Autodesk Fusion 360 part; units mm, degrees
sketch "Skizze8" plane through (0, 0, 0) normal (1, 0, 0) x (0, 1, 0)
  line L0 (-6.5, 80) -> (-16.5, 80)
  line L1 (-16.5, 80) -> (-16.5, -80)
  line L2 (-16.5, -80) -> (-6.5, -80)
  line L3 (-6.5, -80) -> (-6.5, -30)
  line L4 (3.5, -20) -> (25, -20)
  line L5 (35, -10) -> (35, 0)
  line L6 (25, 10) -> (3.5, 10)
  line L7 (105.6778, -5) -> (-37.6639, -5) construction
  line L8 (25, 49.113) -> (25, -113.6091) construction
  line L9 (-6.5, 20) -> (-6.5, 80)
  arc A0 (-6.5, 20) -> (3.5, 10) centre (3.5, 20) ccw
  arc A1 (3.5, -20) -> (-6.5, -30) centre (3.5, -30) ccw
  arc A2 (35, 0) -> (25, 10) centre (25, 0) ccw
  arc A3 (25, -20) -> (35, -10) centre (25, -10) ccw
  circle A4 centre (25, -5) radius 4.15
  point P0 (-6.5, 10)
  dimension "d127" = 80
  dimension "d128" = 80
  dimension "d129" = 5
  dimension "d130" = 31.5
  dimension "d131" = 25
  dimension "d132" = 10
  dimension "d133" = 10
  dimension "d134" = 15
  dimension "d135" = 15
  dimension "d136" = 10
  dimension "d137" = 10
  dimension "d138" = 10
  dimension "d139" = 10
  dimension "d140" = 10
  dimension "d141" = 10
  dimension "d142" = 8.3
extrude "Extrusion8" add sketch "Skizze8" along normal mid plane 40
sketch "Skizze9" plane through (0, 0, 0) normal (0, 0, 1) x (1, 0, 0)
  line L0 (10.1, 40) -> (-10.1, 40)
  line L1 (-10.1, 40) -> (-10.1, -6.5)
  line L2 (-10.1, -6.5) -> (10.1, -6.5)
  line L3 (10.1, -6.5) -> (10.1, 40)
  dimension "d145" = 6.5
  dimension "d146" = 40
  dimension "d147" = 10.1
  dimension "d148" = 10.1
extrude "Extrusion9" cut sketch "Skizze9" along normal mid plane 200
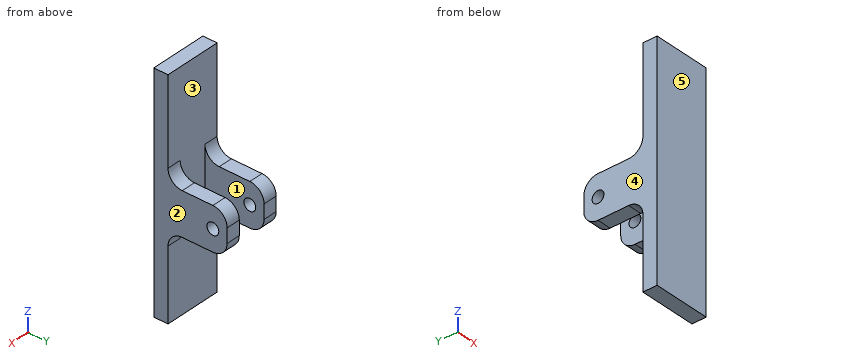
Geometry: final body of the model. Coordinates: model frame, mm. Face numbers are marked on the shaded views. A direction names the side the tool comes from. Round coordinates to 2 decimals unless told otherwise and drop trailing zeros. Write each loop counter-clockwise with the first axis right and the second up, starting at its lowest first coordinate (ties: lowest second). Pieces come first, ordered by that corner, then holes. Notation, with made-up numbers: (46, 30) -> (62, 30) arc R30 ccw to (62, 59) -> close; hole circle Ø6 at (34, -20). An arc over 180 degrees is marked (long way). Use CSV: the item, a comma, the result in double quotes. Start each with the question number.
Q1. Section B-B (y = 11). Return loops of the section in (x, z).
Q2. Section A-A (z = -5). Return loops of the section in (x, y), plus the area to 3 significant figures.
Q3. Section D-D (x = -7.5). Return loops of the section in (y, z), plus the area to 3 significant figures.
Q4. First-contact query: pin 1 Ø11 at (x, y) = (-15, 18.5) entering from +Z; pin 2 Ø7.5 at (y, z) = (25, -5) entering from +X; pin 3 Ø10 at (x, z) = (12, 18) entering from +Y; pin 4 Ø3 at (x, y) = (-16, 10) entering from -Z. Flat tips, straight axial feed; report the tip coordinate or a pass-through.
Q5. Section C-C (x = 11.5). Return loops of the section in (y, z), plus the area to 3 significant figures.
Q6. Pull-direction query (X, two-part tool) for the marked faces 3, 4 and 5; classes: pulls with the +X half, pulls with the -X half, needs draft (parallel to the pull), parting line crosses it, or undercut.
Q7. Reachability of the marked faces 1 and 2 from +Z, -Z, +X, -X, +Y, -Y: full face, straight path, thin tool, end or side. Return the list, or none.
Q8. Line query: L1, parallel to Z at x = -15.5, y = 25; L2, parallel to Y at x = 13, z = -5; L3, parallel to Y at x = -9, z = -6.5. Output: solid intervals per line, ascending.
Result sheet:
1,outline,"(-20, -20) -> (-10.1, -20) -> (-10.1, 10) -> (-20, 10) -> close; (10.1, -20) -> (20, -20) -> (20, 10) -> (10.1, 10) -> close"
2,outline,"(-20, -16.5) -> (20, -16.5) -> (20, 20.85) -> (10.1, 20.85) -> (10.1, -6.5) -> (-10.1, -6.5) -> (-10.1, 20.85) -> (-20, 20.85) -> close; (-20, 29.15) -> (-10.1, 29.15) -> (-10.1, 35) -> (-20, 35) -> close; (10.1, 29.15) -> (20, 29.15) -> (20, 35) -> (10.1, 35) -> close"
2,area,"1,060 mm²"
3,outline,"(-16.5, -80) -> (-6.5, -80) -> (-6.5, 80) -> (-16.5, 80) -> close"
3,area,"1,600 mm²"
4,pin 1,"z = 10"
4,pin 2,"through"
4,pin 3,"y = -3.64"
4,pin 4,"z = -20"
5,outline,"(-16.5, -80) -> (-6.5, -80) -> (-6.5, -30) arc R10 cw to (3.5, -20) -> (25, -20) arc R10 ccw to (35, -10) -> (35, 0) arc R10 ccw to (25, 10) -> (3.5, 10) arc R10 cw to (-6.5, 20) -> (-6.5, 80) -> (-16.5, 80) -> close; hole circle Ø8.3 at (25, -5)"
5,area,"2,790 mm²"
6,face 3,"undercut"
6,face 4,"pulls with the -X half"
6,face 5,"needs draft"
7,face 1,"+Z, -Z, +Y"
7,face 2,"+Z, -Z, +X, +Y, -Y"
8,L1,"-20 to -9.15, -0.85 to 10"
8,L2,"-16.5 to 20.85, 29.15 to 35"
8,L3,"-16.5 to -6.5"
